Can you work these out from the model? Positions are in its coordinate system, mm. Round coordinates to 2 decimals unless told otherwise and drop trailing zeros. Order: outer loops, then holes, each group sorted by start corner. A loop starts at its lowest first (then second) coordinate and runs counter-clockwise, first axis right, second up. Notation, with made-up numbers: (-21, 40.5) -> (9, 40.5) arc R10 ccw to (9, 45.5) -> close; hole circle Ø2 at (47.25, 29). An arc over 180 degrees is marked (long way). One line per item, written item: value.
```python
from build123d import *

# Parameters (mm, degrees)
SKETCH1_R           = 20
SKETCH1_R_2         = 13
BOSS_EXTRUDE1_DEPTH = 8
SKETCH2_W           = 0.6
SKETCH2_H           = 1.3


with BuildPart() as part:
    # Sketch1 → Boss-Extrude1 (new body)
    with BuildSketch(Plane(origin=(0, 0, 0), x_dir=(1, 0, 0), z_dir=(0, 1, 0))):
        with Locations(Location((0, 0, 0), (0, 0, 270))):
            Circle(SKETCH1_R)
        with Locations(Location((0, 0, 0), (0, 0, 270))):
            Circle(SKETCH1_R_2, mode=Mode.SUBTRACT)
    extrude(amount=BOSS_EXTRUDE1_DEPTH)

    # Sketch2 → Cut-Revolve1 (revolve, cut)
    with BuildSketch(Plane(origin=(0, 0, 0), x_dir=(0, 0, -1), z_dir=(1, 0, 0)), mode=Mode.PRIVATE) as cut_revolve1_sk:
        with Locations((13.3, 4.65)):
            Rectangle(SKETCH2_W, SKETCH2_H)
    revolve(cut_revolve1_sk.sketch.rotate(Axis((0, 8, 0), (0, -1, 0)), 180), axis=Axis((0, 8, 0), (0, -1, 0)), mode=Mode.SUBTRACT)


solid = part.part
```
Q1. Please list where these lines run through material, in increasing order: line 1 along X through (y, z) = (4.3, 0); line 2 along X through (y, z) = (6.45, 0); line 3 along Z through (x, y) = (2, 2.5).
Answers below:
line 1: -20 to -13.6, 13.6 to 20
line 2: -20 to -13, 13 to 20
line 3: -19.9 to -12.85, 12.85 to 19.9
Q2. I want a section at D-D on z = -16.5. List the corners of the cut face in (x, y) for me, plus the area to 3 significant figures.
Answers below:
outline: (-11.3, 0) -> (11.3, 0) -> (11.3, 8) -> (-11.3, 8) -> close
area: 181 mm^2
Q3. I want a section at C-C on y = 1. List the corners of the cut face in (x, z) for me.
Answers below:
outline: circle Ø40 at (0, 0); hole circle Ø26 at (0, 0)
Q4. I want a section at B-B on x = 0. List the corners of the cut face in (y, z) for me.
Answers below:
outline: (0, -20) -> (8, -20) -> (8, -13) -> (5.3, -13) -> (5.3, -13.6) -> (4, -13.6) -> (4, -13) -> (0, -13) -> close; (0, 13) -> (4, 13) -> (4, 13.6) -> (5.3, 13.6) -> (5.3, 13) -> (8, 13) -> (8, 20) -> (0, 20) -> close
Q5. I want a section at A-A on z = 0. List the corners of the cut face in (x, y) for me, plus the area to 3 significant figures.
Answers below:
outline: (-20, 0) -> (-13, 0) -> (-13, 4) -> (-13.6, 4) -> (-13.6, 5.3) -> (-13, 5.3) -> (-13, 8) -> (-20, 8) -> close; (13, 0) -> (20, 0) -> (20, 8) -> (13, 8) -> (13, 5.3) -> (13.6, 5.3) -> (13.6, 4) -> (13, 4) -> close
area: 110 mm^2
Q6. We'd pull the mould along Y, two halves only. Please class faces 1 (the face through (-7.91, 1.972, -10.316)), 2 (the face through (-4, 8, 13)), 3 (the face through (13.277, 4.659, -2.948)): released by +Y, released by -Y, zero draft, split by the parting line, or undercut.
Answers below:
face 1: zero draft
face 2: released by +Y
face 3: undercut
Q7. Will these pins go through, and if not, where does the flat tip stop? pin 1 Ø1 at (y, z) = (6.5, 14.5) entering from -X; pin 2 Ø3 at (x, z) = (-13.5, -8) entering from -Y; pin 3 Ø1.5 at (y, z) = (5, -15.5) entering from -X.
Answers below:
pin 1: x = -14.28
pin 2: y = 0
pin 3: x = -13.51
